Input: part model. Units: mm. Frame: model coordinates. Round coordinates to 2 decimals unless told otherwise and drop trailing zeros. Order: outer loops, then holes, each group sorted by start corner. A loop starts at its lowest first (then second) coordinate and runs counter-clockwise, first axis right, second up. Notation, with made-up numbers: (76.5, 18) -> (119.5, 18) arc R15 ccw to (119.5, 41) -> close; hole circle Ø7 at (0, 13.25). An arc over 180 degrees is marked (long way). Use a Markdown table: item, result.
from build123d import *

# Parameters (mm, degrees)
BOSS_EXTRUDE1_DEPTH = 5


with BuildPart() as part:
    # Sketch1 → Boss-Extrude1 (new body)
    with BuildSketch(Plane(origin=(0, 0, 0), x_dir=(1, 0, 0), z_dir=(0, 1, 0))):
        with BuildLine():
            ThreePointArc((0, -56.5), (22.199372282, -51.95611485), (40.828075606, -39.055322843))
            Line((40.828075606, -39.055322843), (40.466765202, -38.709700517))
            ThreePointArc((40.466765202, -38.709700517), (34.104370635, -38.850893215), (33.963177937, -32.488498648))
            Line((33.963177937, -32.488498648), (33.601867534, -32.142876322))
            ThreePointArc((33.601867534, -32.142876322), (18.270279842, -42.76034231), (0, -46.5))
            Line((0, -46.5), (0, -47))
            ThreePointArc((0, -47), (3.181980515, -48.318019485), (4.5, -51.5))
            ThreePointArc((4.5, -51.5), (3.181980515, -54.681980515), (0, -56))
            Line((0, -56), (0, -56.5))
        make_face()
        with BuildLine():
            ThreePointArc((40.828075606, -39.055322843), (52.435847813, -21.041194456), (56.5, 0))
            Line((56.5, 0), (56, 0))
            ThreePointArc((56, 0), (51.5, -4.5), (47, 0))
            Line((47, 0), (46.5, 0))
            ThreePointArc((46.5, 0), (43.155166784, -17.317089243), (33.601867534, -32.142876322))
            Line((33.601867534, -32.142876322), (33.963177937, -32.488498648))
            ThreePointArc((33.963177937, -32.488498648), (38.890818916, -31.422793119), (41.71497157, -35.599099582))
            ThreePointArc((41.71497157, -35.599099582), (41.391278033, -37.274946928), (40.466765202, -38.709700517))
            Line((40.466765202, -38.709700517), (40.828075606, -39.055322843))
        make_face()
        with BuildLine():
            ThreePointArc((56.5, 0), (52.435847813, 21.041194456), (40.828075606, 39.055322843))
            Line((40.828075606, 39.055322843), (40.466765202, 38.709700517))
            ThreePointArc((40.466765202, 38.709700517), (41.391278033, 37.274946928), (41.71497157, 35.599099582))
            ThreePointArc((41.71497157, 35.599099582), (38.890818916, 31.422793119), (33.963177937, 32.488498648))
            Line((33.963177937, 32.488498648), (33.601867534, 32.142876322))
            ThreePointArc((33.601867534, 32.142876322), (43.155166784, 17.317089243), (46.5, 0))
            Line((46.5, 0), (47, 0))
            ThreePointArc((47, 0), (51.5, 4.5), (56, 0))
            Line((56, 0), (56.5, 0))
        make_face()
        with BuildLine():
            ThreePointArc((40.828075606, 39.055322843), (22.199372282, 51.95611485), (0, 56.5))
            Line((0, 56.5), (0, 56))
            ThreePointArc((0, 56), (3.181980515, 54.681980515), (4.5, 51.5))
            ThreePointArc((4.5, 51.5), (3.181980515, 48.318019485), (0, 47))
            Line((0, 47), (0, 46.5))
            ThreePointArc((0, 46.5), (18.270279842, 42.76034231), (33.601867534, 32.142876322))
            Line((33.601867534, 32.142876322), (33.963177937, 32.488498648))
            ThreePointArc((33.963177937, 32.488498648), (34.104370635, 38.850893215), (40.466765202, 38.709700517))
            Line((40.466765202, 38.709700517), (40.828075606, 39.055322843))
        make_face()
        with BuildLine():
            Line((0, 56), (0, 56.5))
            ThreePointArc((0, 56.5), (-22.190806646, 51.959773868), (-40.815196293, 39.068782315))
            Line((-40.815196293, 39.068782315), (-40.453999865, 38.723040879))
            ThreePointArc((-40.453999865, 38.723040879), (-35.526696202, 39.787398082), (-32.703232019, 35.611367951))
            ThreePointArc((-32.703232019, 35.611367951), (-33.027201888, 33.934832134), (-33.952464173, 32.499695023))
            Line((-33.952464173, 32.499695023), (-33.591267745, 32.153953587))
            ThreePointArc((-33.591267745, 32.153953587), (-18.263230248, 42.763353714), (0, 46.5))
            Line((0, 46.5), (0, 47))
            ThreePointArc((0, 47), (-4.5, 51.5), (0, 56))
        make_face()
        with BuildLine():
            Line((-40.453999865, 38.723040879), (-40.815196293, 39.068782315))
            ThreePointArc((-40.815196293, 39.068782315), (-52.43237831, 21.049838592), (-56.5, 0))
            Line((-56.5, 0), (-56, 0))
            ThreePointArc((-56, 0), (-51.5, 4.5), (-47, 0))
            Line((-47, 0), (-46.5, 0))
            ThreePointArc((-46.5, 0), (-43.152311353, 17.324203443), (-33.591267745, 32.153953587))
            Line((-33.591267745, 32.153953587), (-33.952464173, 32.499695023))
            ThreePointArc((-33.952464173, 32.499695023), (-40.314904947, 32.360600105), (-40.453999865, 38.723040879))
        make_face()
        with BuildLine():
            Line((-56, 0), (-56.5, 0))
            ThreePointArc((-56.5, 0), (-51.753754464, -22.667132569), (-38.312428358, -41.525989854))
            Line((-38.312428358, -41.525989854), (-37.973380319, -41.158503218))
            ThreePointArc((-37.973380319, -41.158503218), (-38.229327695, -34.799691148), (-31.870515625, -34.543743772))
            Line((-31.870515625, -34.543743772), (-31.531467586, -34.176257136))
            ThreePointArc((-31.531467586, -34.176257136), (-42.593797922, -18.655250698), (-46.5, 0))
            Line((-46.5, 0), (-47, 0))
            ThreePointArc((-47, 0), (-51.5, -4.5), (-56, 0))
        make_face()
        with BuildLine():
            Line((-37.973380319, -41.158503218), (-38.312428358, -41.525989854))
            ThreePointArc((-38.312428358, -41.525989854), (-20.567347584, -52.623513883), (0, -56.5))
            Line((0, -56.5), (0, -56))
            ThreePointArc((0, -56), (-4.5, -51.5), (0, -47))
            Line((0, -47), (0, -46.5))
            ThreePointArc((0, -46.5), (-16.927109073, -43.30961762), (-31.531467586, -34.176257136))
            Line((-31.531467586, -34.176257136), (-31.870515625, -34.543743772))
            ThreePointArc((-31.870515625, -34.543743772), (-30.799967528, -36.045776653), (-30.421947972, -37.851123495))
            ThreePointArc((-30.421947972, -37.851123495), (-33.11660113, -41.973103939), (-37.973380319, -41.158503218))
        make_face()
    extrude(amount=BOSS_EXTRUDE1_DEPTH)


solid = part.part
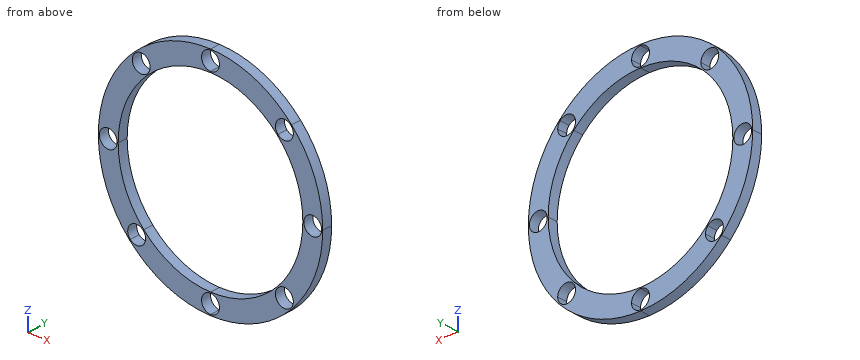
1) Cut plane A-A on x = 51.5. Return loops of the section in (y, z).
Results found:
| item | result |
|---|---|
| outline | (0, -23.24) -> (5, -23.24) -> (5, -4.5) -> (0, -4.5) -> close; (0, 4.5) -> (5, 4.5) -> (5, 23.24) -> (0, 23.24) -> close |
2) Cut plane B-B on z = -27.5. Return loops of the section in (x, y), and give its area (3 significant figures).
Results found:
| item | result |
|---|---|
| outline | (-49.36, 0) -> (-37.5, 0) -> (-37.5, 5) -> (-49.36, 5) -> close; (37.5, 0) -> (49.36, 0) -> (49.36, 5) -> (37.5, 5) -> close |
| area | 119 mm² |
3) Pin query (flat end, axial travel): pin 1 Ø3 at (y, z) = (1, -8.5) entering from -X; pin 2 Ø7 at (x, z) = (51.5, 0) entering from -Y; pin 3 Ø3 at (x, y) = (23.5, 4.5) entering from +Z; pin 4 Ø1 at (x, y) = (-27.5, 1.5) entering from -Z. Return the tip coordinate at first contact, or that it passes through.
Results found:
| item | result |
|---|---|
| pin 1 | stops at x = -56.06 |
| pin 2 | passes through |
| pin 3 | stops at z = 52.04 |
| pin 4 | stops at z = -49.63 |
4) Cut plane C-C on y = 3.45. Count the separate pieces of the cut face and the enclosed holes in it, and give its area (3 significant figures).
Results found:
| item | result |
|---|---|
| separate pieces | 1 |
| enclosed holes | 9 |
| area | 2,730 mm² |
5) Line query: L1, parallel to Z at x = -3.5, y = 2; L2, parallel to X at y = 4.6, z = 34; L3, parallel to X at y = 2.95, z = 31. Output: solid intervals per line, ascending. Write a range as [from, to].
Results found:
| item | result |
|---|---|
| L1 | z = [-56.39, -54.33], [-48.67, -46.37], [46.37, 48.67], [54.33, 56.39] |
| L2 | x = [-45.12, -37.25], [-32.59, -31.72], [31.72, 33.01], [41.42, 45.12] |
| L3 | x = [-47.24, -34.66], [34.66, 47.24] |
